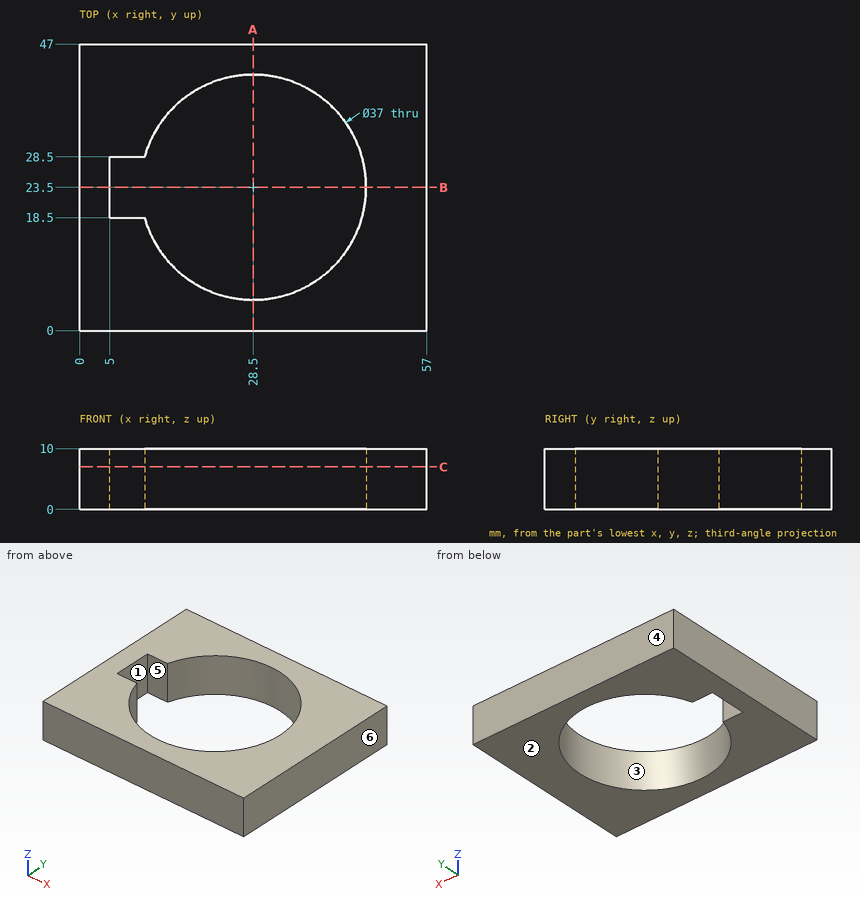
Verification items for this drawing (mm, ordinates from the low corner). A direction names the side the tool comes from. Coordinates: 2 decimals unless noted, no trailing zeros. Loops run counter-clockwise (first coordinate to the right, second up) from the corner with the lowest first, then second, coordinate; pieces in that order, holes last. Notation, with made-up numbers: (78.5, 9) - (119.5, 9) arc R19 cw to (119.5, 17) - close; hole circle Ø6 at (54, 24.5). An arc over 180 degrees is marked (long way). Answer as a JSON object with one key per item and string values.
(1) Cross-section at B-B, the plane y = 23.5. Record the boundary of the cut face in (x, z), then the cut area to 3 significant figures.
Response:
{"outline": "(0, 0) - (5, 0) - (5, 10) - (0, 10) - close; (47, 0) - (57, 0) - (57, 10) - (47, 10) - close", "area": "150 mm²"}
(2) Cross-section at A-A, the plane x = 28.5. Record the boundary of the cut face in (y, z), then the cut area to 3 significant figures.
Response:
{"outline": "(0, 0) - (5, 0) - (5, 10) - (0, 10) - close; (42, 0) - (47, 0) - (47, 10) - (42, 10) - close", "area": "100 mm²"}
(3) Access from +Z, -Z, +X, -X, +Y, -Y to the whole of each face (thin tool, end or side, straight path). Record for the marked faces 1 and 2.
Response:
{"face 1": "+Z, -Z", "face 2": "-Z, +X, -X, +Y, -Y"}
(4) Mould release check, pull along Y, two halves, no side actions. Record for the marked faces 3, 4, 5 and 6: pulls with the +Y half, pulls with the -Y half, needs draft (parallel to the pull), parting line crosses it, or undercut.
Response:
{"face 3": "undercut", "face 4": "pulls with the +Y half", "face 5": "undercut", "face 6": "needs draft"}
(5) Cross-section at C-C, the plane z = 7. Record the boundary of the cut face in (x, y).
Response:
{"outline": "(0, 0) - (57, 0) - (57, 47) - (0, 47) - close; hole (5, 18.5) - (10.69, 18.5) arc R18.5 ccw (long way) to (10.69, 28.5) - (5, 28.5) - close"}
(6) Scan lines: line 1 along X through (y, z) = (23.5, 6.25); line 2 along Y through (x, z) = (29, 8.25); line 3 along X through (y, z) = (7.5, 7.25). Record each from-to range of solid material in increasing order.
Response:
{"line 1": "x = 0 to 5, 47 to 57", "line 2": "y = 0 to 5.01, 41.99 to 47", "line 3": "x = 0 to 19.21, 37.79 to 57"}
